For this review, take the finished solid that the model builds, in its own axes (mm). A direction names the side the tool comes from. Coordinates: 2 decimals unless noted, no trailing zeros. Loops run counter-clockwise (first coordinate to the right, second up) from the corner with the lowest first, then second, coordinate; pieces in that order, holes last. Notation, with made-up numbers: (54, -28.75) -> (75, -28.75) arc R20 ccw to (75, -15.75) -> close; hole circle Ø3 at (54, 46). An arc over 180 degrees is marked (long way). Answer in a Markdown table with one row per item.
from build123d import *

# Parameters (mm, degrees)
EXTRUDE_1_DEPTH      = 48
EXTRUDE_1_DEPTH_BACK = 7
SKETCH_2_R           = 9.9
SKETCH_2_R_2         = 7.9
CUT_EXTRUDE_1_DEPTH  = 2
SKETCH_4_R           = 1.5
CUT_EXTRUDE_2_DEPTH  = 28
CUT_EXTRUDE_3_DEPTH  = 10
SKETCH_7_W           = 3
SKETCH_7_H           = 7
EXTRUDE_3_DEPTH      = 12
CUT_EXTRUDE_4_DEPTH  = 10
CUT_EXTRUDE_START    = 11.8
CUT_EXTRUDE_7_DEPTH  = 2


with BuildPart() as part:
    # Эскиз2 → Бобышка-Вытянуть1 (new, two sides: drawn at the far end of the back side and taken through both)
    # profile 1 of 3: a face of its own
    with BuildSketch(Plane.XY.offset(-EXTRUDE_1_DEPTH_BACK)):
        Circle(SKETCH_2_R)
        Circle(SKETCH_2_R_2, mode=Mode.SUBTRACT)
    # profile 2 of 3: a face of its own
    with BuildSketch(Plane.XY.offset(-EXTRUDE_1_DEPTH_BACK)):
        with BuildLine():
            Line((26, 9.9), (0, 9.9))
            ThreePointArc((0, 9.9), (4.449719092, 8.843641784), (7.949842766, 5.9))
            Line((7.949842766, 5.9), (26, 5.9))
            Line((26, 5.9), (26, 9.9))
        make_face()
    # profile 3 of 3: a face of its own
    with BuildSketch(Plane.XY.offset(-EXTRUDE_1_DEPTH_BACK)):
        with BuildLine():
            ThreePointArc((7.949842766, -5.9), (4.449719092, -8.843641784), (0, -9.9))
            Line((0, -9.9), (26, -9.9))
            Line((26, -9.9), (26, -5.9))
            Line((26, -5.9), (7.949842766, -5.9))
        make_face()
    extrude(amount=EXTRUDE_1_DEPTH + EXTRUDE_1_DEPTH_BACK)

    # Эскиз3 → Вырез-Вытянуть1 (cut)
    with BuildSketch(Plane.XZ.offset(-5.9)):
        Polygon((15.449842766, -1.732050808), (15.449842766, 1.732050808), (12.449842766, 3.464101615), (9.449842766, 1.732050808), (9.449842766, -1.732050808), (12.449842766, -3.464101615), align=None)
        Polygon((12.449842766, 44.464101615), (15.449842766, 42.732050808), (15.449842766, 39.267949192), (12.449842766, 37.535898385), (9.449842766, 39.267949192), (9.449842766, 42.732050808), align=None)
    extrude(amount=-CUT_EXTRUDE_1_DEPTH, mode=Mode.SUBTRACT)

    # Эскиз4 → Вырез-Вытянуть2 (cut)
    with BuildSketch(Plane(origin=(0, 9.9, 0), x_dir=(1, 0, 0), z_dir=(0, 1, 0))):
        with Locations(Location((12.449842766, 0, 0), (0, 0, 270))):
            Circle(SKETCH_4_R)
        with Locations(Location((12.449842766, -41, 0), (0, 0, 270))):
            Circle(SKETCH_4_R)
    extrude(amount=-CUT_EXTRUDE_2_DEPTH, mode=Mode.SUBTRACT)

    # Эскиз5 → Вырез-Вытянуть3 (cut)
    with BuildSketch(Plane(origin=(0, 9.9, 0), x_dir=(1, 0, 0), z_dir=(0, 1, 0))):
        Polygon((23, -38.261238623), (23, -2.738761377), (11.949842766, -9.118572631), (11.949842766, -31.881427369), align=None)
    extrude(amount=-CUT_EXTRUDE_3_DEPTH, mode=Mode.SUBTRACT)

    # Эскиз7 → Бобышка-Вытянуть3 (add)
    with BuildSketch(Plane.XZ.offset(-5.9)):
        with Locations((24.5, 14)):
            Rectangle(SKETCH_7_W, SKETCH_7_H)
        with Locations((24.5, 27)):
            Rectangle(SKETCH_7_W, SKETCH_7_H)
    extrude(amount=EXTRUDE_3_DEPTH)

    # Эскиз8 → Вырез-Вытянуть4 (cut)
    with BuildSketch(Plane.XZ.offset(9.9)):
        Polygon((26, -7), (26, 10.5), (14.207826174, -7), align=None)
        Polygon((26, 48), (26, 31.334606818), (14.207826174, 48), align=None)
        Polygon((23, 22), (9.923665741, 22), (9.923665741, 5.63795963), (18.975811945, 5.63795963), (23, 11.609995999), align=None)
    extrude(amount=-CUT_EXTRUDE_4_DEPTH, mode=Mode.SUBTRACT)

    # Эскиз3<2> → Вырез-Вытянуть7 (cut)
    with BuildSketch(Plane.XZ.offset(-5.9).offset(CUT_EXTRUDE_START)):
        Polygon((15.449842766, 42.732050808), (15.449842766, 39.267949192), (12.449842766, 37.535898385), (9.449842766, 39.267949192), (9.449842766, 42.732050808), (12.449842766, 44.464101615), align=None)
        Polygon((9.449842766, -1.732050808), (12.449842766, -3.464101615), (15.449842766, -1.732050808), (15.449842766, 1.732050808), (12.449842766, 3.464101615), (9.449842766, 1.732050808), align=None)
    extrude(amount=CUT_EXTRUDE_7_DEPTH, mode=Mode.SUBTRACT)


solid = part.part
Item 1: Take a section at A-A, the plane z = 16. State the section outline as (x, y) points, and give its area (3 significant figures).
Worked answers:
| item | result |
|---|---|
| outline | (0, -9.9) -> (9.92, -9.9) -> (9.92, -5.9) -> (7.95, -5.9) arc R9.9 ccw to (7.95, 5.9) -> (11.95, 5.9) -> (11.95, 9.9) -> (0, 9.9) arc R9.9 ccw to start; (23, -9.9) -> (26, -9.9) -> (26, 9.9) -> (23, 9.9) -> close; hole circle Ø15.8 at (0, 0) |
| area | 214 mm² |
Item 2: Take a section at C-C, the plane y = 7. State the section outline as (x, z) points.
Worked answers:
| item | result |
|---|---|
| outline | (-7, -7) -> (-3.66, -7) -> (-3.66, 48) -> (-7, 48) -> close; (3.66, -7) -> (26, -7) -> (26, 48) -> (3.66, 48) -> close; hole (9.45, -1.73) -> (12.45, -3.46) -> (15.45, -1.73) -> (15.45, 1.73) -> (12.45, 3.46) -> (9.45, 1.73) -> close; hole (9.45, 39.27) -> (12.45, 37.54) -> (15.45, 39.27) -> (15.45, 42.73) -> (12.45, 44.46) -> (9.45, 42.73) -> close; hole (11.95, 9.12) -> (23, 2.74) -> (23, 38.26) -> (11.95, 31.88) -> close |
Item 3: Take a section at D-D, the plane z = 0. State the section outline as (x, y) points, and give its area (3 significant figures).
Worked answers:
| item | result |
|---|---|
| outline | (0, -9.9) -> (10.95, -9.9) -> (10.95, -7.9) -> (9.45, -7.9) -> (9.45, -5.9) -> (7.95, -5.9) arc R9.9 ccw to (7.95, 5.9) -> (9.45, 5.9) -> (9.45, 7.9) -> (10.95, 7.9) -> (10.95, 9.9) -> (0, 9.9) arc R9.9 ccw to start; (13.95, -9.9) -> (18.92, -9.9) -> (18.92, -5.9) -> (15.45, -5.9) -> (15.45, -7.9) -> (13.95, -7.9) -> close; (13.95, 7.9) -> (15.45, 7.9) -> (15.45, 5.9) -> (26, 5.9) -> (26, 9.9) -> (13.95, 9.9) -> close; hole circle Ø15.8 at (0, 0) |
| area | 211 mm² |
Item 4: For L1, parallel to Y at x = 9, z = 45; L2, parallel to Y at x = 0, z = 34.5; L3, parallel to Z at x = 13.5, y = -7.5, list the stretches that pass through material, from the lowest coordinate up.
Worked answers:
| item | result |
|---|---|
| L1 | -9.9 to -5.9, -4.12 to 4.12, 5.9 to 9.9 |
| L2 | -9.9 to -7.9, 7.9 to 9.9 |
| L3 | -7 to -2.86, 2.86 to 5.64, 22 to 38.14, 43.86 to 48 |
Item 5: The part is to be moulded in two halves that separate along X. For faces 1 (the flat face through (10, 9.9, 20)), 2 (the flat face through (20.186, -7.928, 39.551)), 3 (the flat face through (14, 7.9, 40)), say which applies: +X half, -X half, draft (parallel to the pull), parting line (faces both ways), or undercut.
Worked answers:
| item | result |
|---|---|
| face 1 | draft |
| face 2 | +X half |
| face 3 | undercut |
Item 6: For faces 4 (the flat face through (11, 7.9, -1)), 5 (the flat face through (20.96, -7.93, 8.58)), 6 (the flat face through (17.552, 7.928, 5.884)), 7 (the flat face through (7, -9.9, 20)), 8 (the flat face through (8, 2, 48)), list the 3-axis set-ups (+Z, -Z, +X, -X, +Y, -Y) from which the entire face can be reached by the end or side of a thin tool; tool diameter is ignored.
Worked answers:
| item | result |
|---|---|
| face 4 | none |
| face 5 | +Y, -Y |
| face 6 | +Y |
| face 7 | +Z, -Z, +X, -X, -Y |
| face 8 | +Z, +X, -X, +Y, -Y |
Item 7: Insertion check: pin 1 (20 mm diameter, centred on x = 16.5, z = 18.5, fed in from +Y); pin 2 (1.5 mm diameter, centred on x = 24, y = -3, fed in from +Z); pin 3 (2.5 mm diameter, centred on x = 12.45, z = 41, fed in from +Y); pin 4 (1.5 mm diameter, centred on y = 6.5, z = 39, fed in from -X). Each pin has a flat end and moves straight along its axis. Give the tip position at first contact, or say it passes through.
Worked answers:
| item | result |
|---|---|
| pin 1 | y = 9.9 |
| pin 2 | z = 30.5 |
| pin 3 | through |
| pin 4 | x = -8.06 |
Item 8: Take a section at B-B, the plane y = 0. State the section outline as (x, z) points.
Worked answers:
| item | result |
|---|---|
| outline | (-9.9, -7) -> (-7.9, -7) -> (-7.9, 48) -> (-9.9, 48) -> close; (7.9, -7) -> (9.9, -7) -> (9.9, 48) -> (7.9, 48) -> close; (23, 10.5) -> (26, 10.5) -> (26, 17.5) -> (23, 17.5) -> close; (23, 23.5) -> (26, 23.5) -> (26, 30.5) -> (23, 30.5) -> close |
